Could you check a few things on this model? Use its own coordinates, in mm. A direction names the side the tool comes from. Give positions to 0.01 mm unless a question says otherwise; leave off trailing zeros. Write each loop counter-clockwise with the first axis right and the second up, starting at its lowest first coordinate (ties: lowest second). Pieces come first, ordered by that corner, then holes. Notation, with made-up numbers: M -2,4.25 L 25,4.25 A20 cw 25,18.25 Z; hole C 28.5,71 d6. An arc over 180 degrees is marked long. One line per item, written item: value.
```python
from build123d import *

# Parameters (mm, degrees)
F0_W      = 5867.4
F0_H      = 7696.2
F1_DEPTH  = 69.135625
F2_W      = 5867.4
F2_H      = 7696.2
F2_W_2    = 5791.2
F2_H_2    = 7620
F3_DEPTH  = 234.95
F4_W      = 38.1
F4_H      = 234.95
F5_DEPTH  = 5863.2060388453
F7_W      = 254
F7_H      = 254
F8_DEPTH  = 7289.8
F9_W      = 184.15
F9_H      = 184.15
F10_DEPTH = 2794
F12_DEPTH = 184.15
F13_W     = 5867.4
F13_H     = 7696.2
F13_W_2   = 5590.8448
F13_H_2   = 7419.6448
F14_DEPTH = 304.085625
F15_W     = 1219.2
F15_H     = 2806.7
F16_DEPTH = 304.8
F17_W     = 368.3
F17_H     = 234.95
F18_DEPTH = 38.1
F19_DEPTH = 38.1
F20_DEPTH = 38.1
F21_SCALE = 0.0114810563


with BuildPart() as f1:
    # F0 (on Top) → F1 (new body)
    with BuildSketch(Plane.XY):
        with Locations((2929.5060388453, -3848.1)):
            Rectangle(F0_W, F0_H)
    extrude(amount=F1_DEPTH)

    # F2 (on face) → F3 (join)
    with BuildSketch(Plane(origin=(0, 0, 0), x_dir=(1, 0, 0), z_dir=(0, 0, -1))):
        with Locations((2929.5060388453, 3848.1)):
            Rectangle(F2_W, F2_H)
        with Locations((2929.5060388453, 3848.1)):
            Rectangle(F2_W_2, F2_H_2, mode=Mode.SUBTRACT)
    extrude(amount=F3_DEPTH)

    # F4 (on Right) → F5 (join, through all)
    with BuildSketch(Plane.YZ):
        with Locations((-425.45, -117.475)):
            Rectangle(F4_W, F4_H)
        with Locations((-831.85, -117.475)):
            Rectangle(F4_W, F4_H)
        with Locations((-1238.25, -117.475)):
            Rectangle(F4_W, F4_H)
        with Locations((-1644.65, -117.475)):
            Rectangle(F4_W, F4_H)
        with Locations((-2051.05, -117.475)):
            Rectangle(F4_W, F4_H)
        with Locations((-2457.45, -117.475)):
            Rectangle(F4_W, F4_H)
        with Locations((-2863.85, -117.475)):
            Rectangle(F4_W, F4_H)
        with Locations((-3270.25, -117.475)):
            Rectangle(F4_W, F4_H)
        with Locations((-3676.65, -117.475)):
            Rectangle(F4_W, F4_H)
        with Locations((-4083.05, -117.475)):
            Rectangle(F4_W, F4_H)
        with Locations((-4489.45, -117.475)):
            Rectangle(F4_W, F4_H)
        with Locations((-4895.85, -117.475)):
            Rectangle(F4_W, F4_H)
        with Locations((-5302.25, -117.475)):
            Rectangle(F4_W, F4_H)
        with Locations((-5708.65, -117.475)):
            Rectangle(F4_W, F4_H)
        with Locations((-6115.05, -117.475)):
            Rectangle(F4_W, F4_H)
        with Locations((-6521.45, -117.475)):
            Rectangle(F4_W, F4_H)
        with Locations((-6927.85, -117.475)):
            Rectangle(F4_W, F4_H)
        with Locations((-7334.25, -117.475)):
            Rectangle(F4_W, F4_H)
    extrude(amount=F5_DEPTH)

    # F7 (on offset) → F8 (join)
    with BuildSketch(Plane(origin=(0, -203.2, 0), x_dir=(-1, 0, 0), z_dir=(0, 1, 0))):
        with Locations((-2929.5060388453, -361.95)):
            Rectangle(F7_W, F7_H)
    extrude(amount=-F8_DEPTH)

    # F9 (on face) → F10 (join)
    with BuildSketch(Plane(origin=(0, 0, -488.95), x_dir=(1, 0, 0), z_dir=(0, 0, -1))):
        with Locations((2929.5060388453, 3848.1)):
            Rectangle(F9_W, F9_H)
    extrude(amount=F10_DEPTH)

    # F11 (on face) → F12 (join, through all)
    with BuildSketch(Plane.YZ.offset(3021.5810388453)):
        Polygon((-3940.175, -838.122572489), (-4289.347572489, -488.95), (-4549.775, -488.95), (-3940.175, -1098.55), align=None)
        Polygon((-3406.852427511, -488.95), (-3756.025, -838.122572489), (-3756.025, -1098.55), (-3146.425, -488.95), align=None)
    extrude(amount=-F12_DEPTH)

    # F13 (on face) → F14 (cut, through all)
    with BuildSketch(Plane.XY.offset(69.135625)):
        with Locations((2929.5060388453, -3848.1)):
            Rectangle(F13_W, F13_H)
        with Locations((2929.5060388453, -3848.1)):
            Rectangle(F13_W_2, F13_H_2, mode=Mode.SUBTRACT)
    extrude(amount=-F14_DEPTH, mode=Mode.SUBTRACT)

    # F15 (on face) → F16 (cut)
    with BuildSketch(Plane.XY.offset(69.135625)):
        with Locations((743.6836388453, -3879.85)):
            Rectangle(F15_W, F15_H)
    extrude(amount=-F16_DEPTH, mode=Mode.SUBTRACT)

    # F17 (on face) → F18 (join)
    with BuildSketch(Plane(origin=(1353.2836388453, 0, 0), x_dir=(0, -1, 0), z_dir=(-1, 0, 0))):
        with Locations((2660.65, -117.475)):
            Rectangle(F17_W, F17_H)
        with Locations((3067.05, -117.475)):
            Rectangle(F17_W, F17_H)
        with Locations((3473.45, -117.475)):
            Rectangle(F17_W, F17_H)
        with Locations((3879.85, -117.475)):
            Rectangle(F17_W, F17_H)
        with Locations((4286.25, -117.475)):
            Rectangle(F17_W, F17_H)
        with Locations((4692.65, -117.475)):
            Rectangle(F17_W, F17_H)
        with Locations((5099.05, -117.475)):
            Rectangle(F17_W, F17_H)
    extrude(amount=-F18_DEPTH)

    # F19 (add): a face of the model
    f19_faces = [f1.faces().sort_by_distance(p)[0] for p in [
        (2929.5060388453, -5321.3, -117.475),
    ]]
    extrude(f19_faces, amount=F19_DEPTH)

    # F20 (add): a face of the model
    f20_faces = [f1.faces().sort_by_distance(p)[0] for p in [
        (2929.5060388453, -2438.4, -117.475),
    ]]
    extrude(f20_faces, amount=F20_DEPTH)


with BuildPart() as f1_1:
    # F21: moved
    add(f1.part.scale(F21_SCALE))


solid = f1_1.part
```
1) If we section it at B-B, the plane z = -7: Write out the boundary of the cut face in (x, y), then the cut area to 3 significant figures.
Outcome:
outline: M 32.58,-50.85 L 34.69,-50.85 L 34.69,-47.86 L 32.58,-47.86 Z; M 32.58,-45.24 L 34.69,-45.24 L 34.69,-43.12 L 32.58,-43.12 Z; M 32.58,-40.5 L 34.69,-40.5 L 34.69,-37.51 L 32.58,-37.51 Z
area: 17.1 mm^2
2) I'm going to push flat-ended pins straight in: pin 1 (0.8 mm diameter, centred on x = 47, z = -1, fed in from -Y); pin 2 (6 mm diameter, centred on x = 22.5, z = -8, fed in from -Y); pin 3 (5 mm diameter, centred on y = -47, z = -15, fed in from -X); pin 4 (0.9 mm diameter, centred on x = 33, z = -4, fed in from +Y). Where does each tip first touch, or does it pass through?
Outcome:
pin 1: stops at y = -84.42
pin 2: passes through
pin 3: stops at x = 32.58
pin 4: stops at y = -2.33
3) If we section it at C-C, the plane z = -31.5: Write out the boundary of the cut face in (x, y), then the cut area to 3 significant figures.
Outcome:
outline: M 32.58,-45.24 L 34.69,-45.24 L 34.69,-43.12 L 32.58,-43.12 Z
area: 4.47 mm^2
4) We'd pull the mould along Y, two halves only. Please class faces 1 (the face through (15.975, -59, -1)), 2 (the face through (33.65, -48.79, -9.06)), 3 (the face through (35.092, -44, -4)): pulls with the +Y half, pulls with the -Y half, needs draft (parallel to the pull), parting line crosses it, or undercut.
Outcome:
face 1: undercut
face 2: pulls with the -Y half
face 3: needs draft
5) Please list where these lines run through material, in increasing order: L1, parallel to Z at x = 20.5, y = -61.5; L2, parallel to X at y = -18.5, z = -4; L3, parallel to X at y = -50.5, z = -6.5. Write a range as from..to.
Outcome:
L1: z = -2.7..0.79
L2: x = 32.18..35.09
L3: x = 32.58..34.69
6) On a 3-axis mill with a long thin cutter (end or side, diameter ignored), from which of +Z, -Z, +X, -X, +Y, -Y can I reach the whole of each face in a straight line? I mean faces 4 (the face through (15.975, -40, -1)), 5 (the face through (34, -77, -2.697)), 6 (the face through (34, -54, -2.697)), 7 (the face through (1.539, -17.1, 0.2)). Say none if no direction works.
Outcome:
face 4: -Z, +X
face 5: +X, -X
face 6: +X
face 7: +Z, -Z, -X, +Y, -Y
7) If we section it at A-A, the plane y = -41: Write out the boundary of the cut face in (x, z).
Outcome:
outline: M 15.54,-2.7 L 15.97,-2.7 L 15.97,0 L 65.73,0 L 65.73,0.79 L 15.54,0.79 Z; M 32.18,-5.61 L 35.09,-5.61 L 35.09,-2.7 L 32.18,-2.7 Z; M 32.58,-10.49 L 34.69,-10.49 L 34.69,-7.5 L 32.58,-7.5 Z
